from build123d import *

# Parameters (mm, degrees)
SKETCH_1_W             = 57
SKETCH_1_H             = 57
EXTRUDE_1_DEPTH        = 25
SKETCH_2_R             = 19.05
CUT_EXTRUDE_1_DEPTH    = 51
SKETCH_3_W             = 40
SKETCH_3_H             = 35
CUT_EXTRUDE_2_DEPTH    = 32
CHAMFER_1_SIZE         = 5
HOLE_WIZARD_M4_1_D     = 3.3
HOLE_WIZARD_M4_1_DEPTH = 18.5
HOLE_WIZARD_M4_1_TIP   = 0.991420021
FILLET_1_R             = 5
HOLE_WIZARD_M3_1_D     = 2.5
HOLE_WIZARD_M3_1_DEPTH = 10
HOLE_WIZARD_M3_1_TIP   = 0.751075774
HOLE_WIZARD_M4_2_D     = 3.3
HOLE_WIZARD_M4_2_DEPTH = 18.5
HOLE_WIZARD_M4_2_TIP   = 0.991420021


with BuildPart() as part:
    # 草图1 → 凸台-拉伸1 (new body, symmetric)
    with BuildSketch(Plane.XY):
        Rectangle(SKETCH_1_W, SKETCH_1_H)
    extrude(amount=EXTRUDE_1_DEPTH, both=True)

    # 草图2 → 切除-拉伸1 (cut, through all)
    with BuildSketch(Plane(origin=(0, 0, -25), x_dir=(-1, 0, 0), z_dir=(0, 0, -1))):
        Circle(SKETCH_2_R)
    extrude(amount=-CUT_EXTRUDE_1_DEPTH, mode=Mode.SUBTRACT)

    # 草图3 → 切除-拉伸2 (cut)
    with BuildSketch(Plane(origin=(-28.5, 0, 0), x_dir=(0, 0, -1), z_dir=(1, 0, 0))):
        Rectangle(SKETCH_3_W, SKETCH_3_H)
    extrude(amount=CUT_EXTRUDE_2_DEPTH, mode=Mode.SUBTRACT)

    # 倒角1
    chamfer_1_edges = [part.edges().sort_by_distance(p)[0] for p in [
        (28.5, -28.5, 0),
        (-28.5, -28.5, 0),
        (-28.5, 28.5, 0),
        (28.5, 28.5, 0),
    ]]
    chamfer(chamfer_1_edges, length=CHAMFER_1_SIZE)

    # M4 螺纹孔1
    with Locations(Plane(origin=(0, 0, -25), x_dir=(-1, 0, 0), z_dir=(0, 0, -1))):
        with Locations((-23.5, 23.5), (23.5, 23.5), (23.5, -23.5), (-23.5, -23.5)):
            Hole(HOLE_WIZARD_M4_1_D / 2, depth=HOLE_WIZARD_M4_1_DEPTH)
            with Locations((0, 0, -(HOLE_WIZARD_M4_1_DEPTH + HOLE_WIZARD_M4_1_TIP / 2))):  # 118° drill point
                Cone(0, HOLE_WIZARD_M4_1_D / 2, HOLE_WIZARD_M4_1_TIP, mode=Mode.SUBTRACT)

    # 圆角1
    fillet_1_edges = [part.edges().sort_by_distance(p)[0] for p in [
        (-18.013392751, -17.5, -20),
        (-18.013392751, 17.5, -20),
        (-18.013392751, 17.5, 20),
        (-18.013392751, -17.5, 20),
    ]]
    fillet(fillet_1_edges, radius=FILLET_1_R)

    # M3 螺纹孔1
    with Locations(Plane.ZY.offset(28.5)):
        with Locations((21, 19), (-21, 19), (-21, -19), (21, -19)):
            Hole(HOLE_WIZARD_M3_1_D / 2, depth=HOLE_WIZARD_M3_1_DEPTH)
            with Locations((0, 0, -(HOLE_WIZARD_M3_1_DEPTH + HOLE_WIZARD_M3_1_TIP / 2))):  # 118° drill point
                Cone(0, HOLE_WIZARD_M3_1_D / 2, HOLE_WIZARD_M3_1_TIP, mode=Mode.SUBTRACT)

    # M4 螺纹孔2
    with Locations(Plane.XY.offset(25)):
        with Locations((23.5, 23.5), (-23.5, 23.5), (-23.5, -23.5), (23.5, -23.5)):
            Hole(HOLE_WIZARD_M4_2_D / 2, depth=HOLE_WIZARD_M4_2_DEPTH)
            with Locations((0, 0, -(HOLE_WIZARD_M4_2_DEPTH + HOLE_WIZARD_M4_2_TIP / 2))):  # 118° drill point
                Cone(0, HOLE_WIZARD_M4_2_D / 2, HOLE_WIZARD_M4_2_TIP, mode=Mode.SUBTRACT)


solid = part.part
The model under review builds one solid part; all positions refer to its coordinate system, in mm. A direction names the side the tool comes from. Round coordinates to 2 decimals unless told otherwise and drop trailing zeros. Loops run counter-clockwise (first coordinate to the right, second up) from the corner with the lowest first, then second, coordinate; pieces in that order, holes last. Notation, with made-up numbers: M -24,54.25 L 10,54.25 A25 ccw 10,93.25 Z; hole C 0,42.25 d7. An arc over 180 degrees is marked long. Answer as CSV lines item,"result".
1. We need section B-B (y = -8). Give the boundary of the cut face in (x, z), plus the area to 3 significant figures.
Outcome:
outline,"M -28.5,-25 L -17.29,-25 L -17.29,-20 L -28.5,-20 Z; M -28.5,20 L -17.29,20 L -17.29,25 L -28.5,25 Z; M 17.29,-25 L 28.5,-25 L 28.5,25 L 17.29,25 Z"
area,"673 mm2"
2. For faces 1 (the face through (-24.716, 24.615, -15.62)), 2 (the face through (-20.2, -16.07, 18.5)), 3 (the face through (24.716, -22.385, 15.62)), list the 3-axis set-ups (+Z, -Z, +X, -X, +Y, -Y) from which the entire face can be reached by the end or side of a thin tool; tool diameter is ignored.
Outcome:
face 1,"-Z"
face 2,"-X"
face 3,"+Z"
3. Insertion check: pin 1 Ø8 at (x, y) = (12, 1) entering from -Z; pin 2 Ø2 at (y, z) = (-19, 21) entering from -X; pin 3 Ø2.5 at (x, y) = (23.5, 23.5) entering from -Z; pin 4 Ø3 at (x, y) = (-23.5, 23.5) entering from -Z. Each pin has a flat end and moves straight along its axis. Give the tip position at first contact, or say it passes through.
Outcome:
pin 1,"passes through"
pin 2,"stops at x = -18.35"
pin 3,"stops at z = -6.26"
pin 4,"stops at z = -6.41"
4. Draft analysis for pull direction Z (two halves, no side actions). For faces 4 (the face through (-23.35, 23.74, 5.68)), 5 (the face through (24.716, 24.615, 15.62)), 6 (the face through (-23.43, 18.521, 19.845)), state which applies: pulls with the +Z half, pulls with the -Z half, needs draft (parallel to the pull), parting line crosses it, or undercut.
Outcome:
face 4,"pulls with the +Z half"
face 5,"needs draft"
face 6,"undercut"
5. We need section D-D (z = -12.5). Give the boundary of the cut face in (x, y).
Outcome:
outline,"M -28.5,-23.5 L -23.5,-28.5 L 23.5,-28.5 L 28.5,-23.5 L 28.5,23.5 L 23.5,28.5 L -23.5,28.5 L -28.5,23.5 L -28.5,17.5 L -7.53,17.5 A19.05 cw long -7.53,-17.5 L -28.5,-17.5 Z; hole C -23.5,-23.5 d3.3; hole C -23.5,23.5 d3.3; hole C 23.5,-23.5 d3.3; hole C 23.5,23.5 d3.3"
6. We need section A-A (x = 0). Give the boundary of the cut face in (y, z), plus the area to 3 significant figures.
Outcome:
outline,"M -28.5,-25 L -19.05,-25 L -19.05,25 L -28.5,25 Z; M 19.05,-25 L 28.5,-25 L 28.5,25 L 19.05,25 Z"
area,"945 mm2"
7. We need section C-C (z = -2.5). Give the boundary of the cut face in (x, y), plus the area to 3 significant figures.
Outcome:
outline,"M -28.5,-23.5 L -23.5,-28.5 L 23.5,-28.5 L 28.5,-23.5 L 28.5,23.5 L 23.5,28.5 L -23.5,28.5 L -28.5,23.5 L -28.5,17.5 L -7.53,17.5 A19.05 cw long -7.53,-17.5 L -28.5,-17.5 Z"
area,"1,620 mm2"
8. To check wall thickness, follow L1, parallel to Y at x = -21.5, z = 21; L2, parallel to Y at x = 23.5, z = 12.5; L3, parallel to Y at x = -23.5, z = 11. State the ranges of each line that lie inside material, in increasing order. Write a range as [from, to].
Outcome:
L1,"y = [-28.5, -20.25], [-17.75, 17.75], [20.25, 28.5]"
L2,"y = [-28.5, -25.15], [-21.85, 21.85], [25.15, 28.5]"
L3,"y = [-28.5, -25.15], [-21.85, -17.5], [17.5, 21.85], [25.15, 28.5]"
